from build123d import *

# Parameters (mm, degrees)
SKETCH3_W           = 120.6
SKETCH3_H           = 124
BOSS_EXTRUDE3_DEPTH = 44
SKETCH9_W           = 116.6
SKETCH9_H           = 124
CUT_EXTRUDE2_DEPTH  = 42
SKETCH10_W          = 120.6
SKETCH10_H          = 2.5
CUT_EXTRUDE3_DEPTH  = 42
SKETCH11_W          = 120.6
SKETCH11_H          = 2.5
CUT_EXTRUDE4_DEPTH  = 42
SKETCH12_R          = 1.55
CUT_EXTRUDE5_DEPTH  = 124.6


with BuildPart() as part:
    # Sketch3 → Boss-Extrude3 (new body)
    with BuildSketch(Plane(origin=(0, 0, 0), x_dir=(1, 0, 0), z_dir=(0, 1, 0))):
        Rectangle(SKETCH3_W, SKETCH3_H)
    extrude(amount=BOSS_EXTRUDE3_DEPTH)

    # Sketch9 → Cut-Extrude2 (cut, through all)
    with BuildSketch(Plane(origin=(0, 3, 0), x_dir=(1, 0, 0), z_dir=(0, 1, 0))):
        Rectangle(SKETCH9_W, SKETCH9_H)
    extrude(amount=CUT_EXTRUDE2_DEPTH, mode=Mode.SUBTRACT)

    # Sketch10 → Cut-Extrude3 (cut, through all)
    with BuildSketch(Plane(origin=(0, 3, 0), x_dir=(1, 0, 0), z_dir=(0, 1, 0))):
        with Locations((0, 60.75)):
            Rectangle(SKETCH10_W, SKETCH10_H)
    extrude(amount=CUT_EXTRUDE3_DEPTH, mode=Mode.SUBTRACT)

    # Sketch11 → Cut-Extrude4 (cut, through all)
    with BuildSketch(Plane(origin=(0, 3, 0), x_dir=(1, 0, 0), z_dir=(0, 1, 0))):
        with Locations((0, -60.75)):
            Rectangle(SKETCH11_W, SKETCH11_H)
    extrude(amount=CUT_EXTRUDE4_DEPTH, mode=Mode.SUBTRACT)

    # Sketch12 → Cut-Extrude5 (cut, through all)
    with BuildSketch(Plane.ZY.offset(63.3)):
        with Locations((-22.5, 38)):
            Circle(SKETCH12_R)
        with Locations((17.5, 38)):
            Circle(SKETCH12_R)
    extrude(amount=-CUT_EXTRUDE5_DEPTH, mode=Mode.SUBTRACT)


solid = part.part
Verification items for the finished model (mm, model axes). A direction names the side the tool comes from. Round coordinates to 2 decimals unless told otherwise and drop trailing zeros. Loops run counter-clockwise (first coordinate to the right, second up) from the corner with the lowest first, then second, coordinate; pieces in that order, holes last. Notation, with made-up numbers: (-14.75, -30) - (-3.75, -30) arc R17 ccw to (-3.75, -20) - close; hole circle Ø5 at (44, 30). An arc over 180 degrees is marked (long way). Answer in a Markdown table with one row per item. Add a question column.
Q1. Section check C-C on z = -4. Enter the section's corners in (x, y).
Q2. Tool access check on faces 1 (the face through (-58.3, 23, 1)), 2 (the face through (60.3, 22, 1)). Record the directions out of +Z, -Z, +X, -X, +Y, -Y that give a thin tool (end or side, any length) a straight path to the whole face; none if there is none.
Q3. Material ranges on line 1 (Y direction, x = 58.95, z = -22.5); line 2 (X direction, y = 34.5, z = -48); line 3 (Y direction, x = 2, z = -56), recorded low to high.
Q4. Section check D-D on y = 16.5. Enter the section's corners in (x, z), plus the area to 3 significant figures.
Q5. Section check B-B on z = 17.5. Enter the section's corners in (x, y).
Q6. Release check for a two-part mould opening along X. For faces 3 (the face through (-60.3, 22, 1)), 4 (the face through (58.3, 23, 1)), 5 (the face through (59.286, 36.487, 17.164)) record: pulls with the +X half, pulls with the -X half, needs draft (parallel to the pull), parting line crosses it, or undercut.
Q7. Section check A-A on y = 38. Enter the section's corners in (x, z), plus the area to 3 significant figures.
Q8. Gauge pin test, flat ends, axial feed: pin 1 (1.9 mm diameter, centred on y = 38, z = 17.5, fed in from -X); pin 2 (1.6 mm diameter, centred on x = 59, y = 20, fed in from -Z); pin 3 (2 mm diameter, centred on x = -21.5, z = -40, fed in from -Y); pin 4 (2 mm diameter, centred on x = 59.5, y = 24.5, fed in from +Z). Record the tip position at first contact, or that the pin passes through.
Found:
| question | item | result |
|---|---|---|
| 1 | outline | (-60.3, 0) - (60.3, 0) - (60.3, 44) - (58.3, 44) - (58.3, 3) - (-58.3, 3) - (-58.3, 44) - (-60.3, 44) - close |
| 2 | face 1 | +Z, -Z, +Y |
| 2 | face 2 | +Z, -Z, +X, +Y, -Y |
| 3 | line 1 | y = 0 to 36.45, 39.55 to 44 |
| 3 | line 2 | x = -60.3 to -58.3, 58.3 to 60.3 |
| 3 | line 3 | y = 0 to 3 |
| 4 | outline | (-60.3, -59.5) - (-58.3, -59.5) - (-58.3, 59.5) - (-60.3, 59.5) - close; (58.3, -59.5) - (60.3, -59.5) - (60.3, 59.5) - (58.3, 59.5) - close |
| 4 | area | 476 mm² |
| 5 | outline | (-60.3, 0) - (60.3, 0) - (60.3, 36.45) - (58.3, 36.45) - (58.3, 3) - (-58.3, 3) - (-58.3, 36.45) - (-60.3, 36.45) - close; (-60.3, 39.55) - (-58.3, 39.55) - (-58.3, 44) - (-60.3, 44) - close; (58.3, 39.55) - (60.3, 39.55) - (60.3, 44) - (58.3, 44) - close |
| 6 | face 3 | pulls with the -X half |
| 6 | face 4 | undercut |
| 6 | face 5 | needs draft |
| 7 | outline | (-60.3, -59.5) - (-58.3, -59.5) - (-58.3, -24.05) - (-60.3, -24.05) - close; (-60.3, -20.95) - (-58.3, -20.95) - (-58.3, 15.95) - (-60.3, 15.95) - close; (-60.3, 19.05) - (-58.3, 19.05) - (-58.3, 59.5) - (-60.3, 59.5) - close; (58.3, -59.5) - (60.3, -59.5) - (60.3, -24.05) - (58.3, -24.05) - close; (58.3, -20.95) - (60.3, -20.95) - (60.3, 15.95) - (58.3, 15.95) - close; (58.3, 19.05) - (60.3, 19.05) - (60.3, 59.5) - (58.3, 59.5) - close |
| 7 | area | 451 mm² |
| 8 | pin 1 | passes through |
| 8 | pin 2 | stops at z = -59.5 |
| 8 | pin 3 | stops at y = 0 |
| 8 | pin 4 | stops at z = 59.5 |
